The drawing under review shows one solid part. Ordinate dimensions are in mm from its lowest x, y, z. A direction names the side the tool comes from. Round coordinates to 2 decimals unless told otherwise and drop trailing zeros. Order: outer loops, then holes, each group sorted by start corner. A loop starts at its lowest first (then second) coordinate and runs counter-clockwise, first axis right, second up. Notation, with made-up numbers: (16.25, 47.5) -> (25.25, 47.5) arc R27 ccw to (25.25, 63.5) -> close; hole circle Ø9 at (65.25, -35.75). An arc over 180 degrees is marked (long way). Use a Markdown table: item, result. Add a question column.
1) Consider section B-B (y = 8.75). State the section outline as (x, z) points, plus the area to 3 significant figures.
2) Machinability: for the marked faces 5, 6 and 7, which of the approach directions +Z, -Z, +X, -X, +Y, -Y give a long, thin tool a straight path to every point of the face, cutting with its end or side? Answer none if there is none.
3) Consider section D-D (z = 12.7). State the section outline as (x, y) points.
4) Clearance check with flat-ended pins moving along their axes: P1, Ø3.5, axis at y = 11.83, z = 3.3, coming from the -X side; P2, Ø2, axis at y = 3.5, z = 5.5, coming from the +X side; P3, Ø4, axis at x = 4, z = 7.5, coming from the +Y side; P4, Ø2.5, axis at x = 26, z = 8, coming from the -Y side. State where each tip first meets the part, or that it passes through.
5) Wall thickness on line 1 along X through (y, z) = (0.45, 8); line 2 along X through (y, z) = (7.5, 9.25); line 3 along Y through (x, z) = (19.1, 3.3): over which ranges is each line inside the solid? List them lowest first. Write a range as [from, to].
6) Consider section A-A (z = 8). State the section outline as (x, y) points.
7) Draft analysis for pull direction X (two halves, no side actions). For the marked faces 1, 2, 3 and 4, state which applies: pulls with the +X half, pulls with the -X half, needs draft (parallel to the pull), parting line crosses it, or undercut.
8) Consider section C-C (x = 26). State the section outline as (y, z) points, plus the area to 3 significant figures.
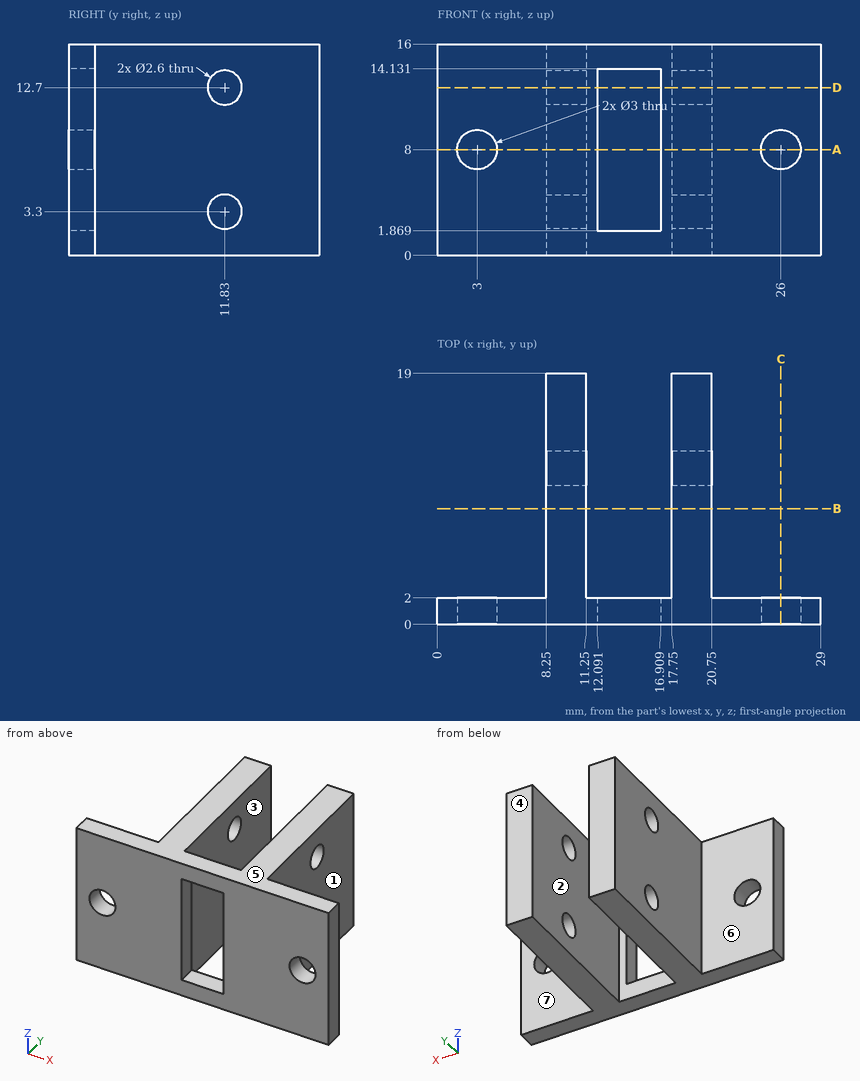
Results list:
| question | item | result |
|---|---|---|
| 1 | outline | (8.25, 0) -> (11.25, 0) -> (11.25, 16) -> (8.25, 16) -> close; (17.75, 0) -> (20.75, 0) -> (20.75, 16) -> (17.75, 16) -> close |
| 1 | area | 96.0 mm2 |
| 2 | face 5 | +Z, +X, -X, +Y, -Y |
| 2 | face 6 | +Z, -Z, -X, +Y |
| 2 | face 7 | +Z, -Z, +X, +Y |
| 3 | outline | (0, 0) -> (12.09, 0) -> (12.09, 2) -> (11.25, 2) -> (11.25, 10.53) -> (8.25, 10.53) -> (8.25, 2) -> (0, 2) -> close; (8.25, 13.13) -> (11.25, 13.13) -> (11.25, 19) -> (8.25, 19) -> close; (16.91, 0) -> (29, 0) -> (29, 2) -> (20.75, 2) -> (20.75, 10.53) -> (17.75, 10.53) -> (17.75, 2) -> (16.91, 2) -> close; (17.75, 13.13) -> (20.75, 13.13) -> (20.75, 19) -> (17.75, 19) -> close |
| 4 | P1 | x = 8.25 |
| 4 | P2 | x = 20.75 |
| 4 | P3 | y = 2 |
| 4 | P4 | through |
| 5 | line 1 | [0, 1.5], [4.5, 12.09], [16.91, 24.5], [27.5, 29] |
| 5 | line 2 | [8.25, 11.25], [17.75, 20.75] |
| 5 | line 3 | [0, 10.53], [13.13, 19] |
| 6 | outline | (0, 0) -> (1.5, 0) -> (1.5, 2) -> (0, 2) -> close; (4.5, 0) -> (12.09, 0) -> (12.09, 2) -> (11.25, 2) -> (11.25, 19) -> (8.25, 19) -> (8.25, 2) -> (4.5, 2) -> close; (16.91, 0) -> (24.5, 0) -> (24.5, 2) -> (20.75, 2) -> (20.75, 19) -> (17.75, 19) -> (17.75, 2) -> (16.91, 2) -> close; (27.5, 0) -> (29, 0) -> (29, 2) -> (27.5, 2) -> close |
| 7 | face 1 | pulls with the +X half |
| 7 | face 2 | undercut |
| 7 | face 3 | undercut |
| 7 | face 4 | needs draft |
| 8 | outline | (0, 0) -> (2, 0) -> (2, 6.5) -> (0, 6.5) -> close; (0, 9.5) -> (2, 9.5) -> (2, 16) -> (0, 16) -> close |
| 8 | area | 26.0 mm2 |
